Input: part model. Units: mm. Frame: model coordinates. A direction names the side the tool comes from. Give positions to 0.01 mm unless a question says otherwise; leave off trailing zeros. Loops run counter-clockwise (first coordinate to the right, second up) from the corner with the lowest first, then second, coordinate; pieces in that order, holes last. Notation, with made-up numbers: (51, -12) - (107, -12) arc R23 ccw to (107, 16) - close; hole circle Ø4 at (72, 40). An arc over 180 degrees is marked (long way). Answer as a JSON object with one key per item and string values. Group by question number.
(1) Section query A-A (z = -1.25). Return loops of the section in (x, y), plus the area to 3 significant figures.
(2) Section query B-B (x = 12). Return loops of the section in (y, z), plus the area to 3 significant figures.
(3) Mould query, pull axis X, two halves, no side actions, for faces 4 (the flat face through (-19.05, -3, -0.02)), 5 (the flat face through (12, -5, 0)), 6 (the cylindrical face through (19, -4, -4)), 7 (the cylindrical face through (-15, -1, 4)). Classes: +X half, -X half, draft (parallel to the pull), parting line (faces both ways), or undercut.
(4) Pin query (flat end, axial travel): P1, Ø0.9, axis at y = -2, z = -0.5, coming from the +X side; P2, Ø3.5, axis at y = -1, z = 0.5, coming from the -X side; P3, Ø5, axis at x = -13, z = 2, coming from the -Y side. Return the tip coordinate at first contact, or that it passes through.
(5) Access query for faces 1 (the flat face through (14.95, -3, -0.02)), 2 (the flat face through (0, -5, 0)), 3 (the flat face through (-19.5, -4, 0)). Directions: +Z, -Z, +X, -X, +Y, -Y. A direction counts if a zero-diameter tool reaches every point of the face in a straight line with its end or side. Return the directions, or none.
(6) Section query C-C (z = 2). Return loops of the section in (x, y).
(7) Section query D-D (x = -1.5). Return loops of the section in (y, z).
(8) Material intervals for L1, parallel to X at y = -1.25, z = -2.25; L2, parallel to Y at x = 7, z = 4.5; L3, parallel to X at y = -0.75, z = -3.25, sorted ascending.
```python
from build123d import *

# Parameters (mm, degrees)
BOSS_EXTRU_2_DEPTH      = 5
BOSS_EXTRU_7_DEPTH      = 7
ESQUISSE1_13_W          = 0.6
ESQUISSE1_13_H          = 2.5
ENL_V_MAT_EXTRU_3_DEPTH = 3
ESQUISSE1_16_W          = 0.6
ESQUISSE1_16_H          = 2.5
ENL_V_MAT_EXTRU_4_DEPTH = 3


with BuildPart() as part:
    # Esquisse1 → Boss.-Extru.2 (new body)
    with BuildSketch(Plane(origin=(0, 0, 0), x_dir=(1, 0, 0), z_dir=(0, 1, 0))):
        with BuildLine():
            Line((-17, -5), (17, -5))
            ThreePointArc((17, -5), (18.767766953, -4.267766953), (19.5, -2.5))
            Line((19.5, -2.5), (19.5, 2.5))
            ThreePointArc((19.5, 2.5), (18.767766953, 4.267766953), (17, 5))
            Line((17, 5), (-17, 5))
            ThreePointArc((-17, 5), (-18.767766953, 4.267766953), (-19.5, 2.5))
            Line((-19.5, 2.5), (-19.5, -2.5))
            ThreePointArc((-19.5, -2.5), (-18.767766953, -4.267766953), (-17, -5))
        make_face()
    extrude(amount=-BOSS_EXTRU_2_DEPTH)

    # Esquisse1_9 → Boss.-Extru.7 (add)
    with BuildSketch(Plane(origin=(0, 0, 0), x_dir=(1, 0, 0), z_dir=(0, 1, 0))):
        with BuildLine():
            ThreePointArc((-5, 0), (-3.535533906, -3.535533906), (0, -5))
            ThreePointArc((0, -5), (3.535533906, -3.535533906), (5, 0))
            Line((5, 0), (3.5, 0))
            ThreePointArc((3.5, 0), (0, -3.5), (-3.5, 0))
            Line((-3.5, 0), (-5, 0))
        make_face()
        with BuildLine():
            Line((3.5, 0), (5, 0))
            ThreePointArc((5, 0), (3.535533906, 3.535533906), (0, 5))
            ThreePointArc((0, 5), (-3.535533906, 3.535533906), (-5, 0))
            Line((-5, 0), (-3.5, 0))
            ThreePointArc((-3.5, 0), (0, 3.5), (3.5, 0))
        make_face()
    extrude(amount=-BOSS_EXTRU_7_DEPTH)

    # Esquisse1_13 → Enl_v. mat.-Extru.3 (cut)
    with BuildSketch(Plane(origin=(0, 0, 0), x_dir=(1, 0, 0), z_dir=(0, 1, 0))):
        with BuildLine():
            ThreePointArc((17, 5), (15.232233047, 4.267766953), (14.5, 2.5))
            Line((14.5, 2.5), (15.1, 2.5))
            ThreePointArc((15.1, 2.5), (15.656497116, 3.843502884), (17, 4.4))
            Line((17, 4.4), (17, 5))
        make_face()
        with BuildLine():
            ThreePointArc((19.5, 2.5), (18.767766953, 4.267766953), (17, 5))
            Line((17, 5), (17, 4.4))
            ThreePointArc((17, 4.4), (18.343502884, 3.843502884), (18.9, 2.5))
            Line((18.9, 2.5), (19.5, 2.5))
        make_face()
        with Locations((19.2, 1.25)):
            Rectangle(ESQUISSE1_13_W, ESQUISSE1_13_H)
        with Locations((19.2, -1.25)):
            Rectangle(ESQUISSE1_13_W, ESQUISSE1_13_H)
        with BuildLine():
            Line((17, -4.4), (17, -5))
            ThreePointArc((17, -5), (18.767766953, -4.267766953), (19.5, -2.5))
            Line((19.5, -2.5), (18.9, -2.5))
            ThreePointArc((18.9, -2.5), (18.343502884, -3.843502884), (17, -4.4))
        make_face()
        with BuildLine():
            ThreePointArc((14.5, -2.5), (15.232233047, -4.267766953), (17, -5))
            Line((17, -5), (17, -4.4))
            ThreePointArc((17, -4.4), (15.656497116, -3.843502884), (15.1, -2.5))
            Line((15.1, -2.5), (14.5, -2.5))
        make_face()
        with Locations((14.8, -1.25)):
            Rectangle(ESQUISSE1_13_W, ESQUISSE1_13_H)
        with Locations((14.8, 1.25)):
            Rectangle(ESQUISSE1_13_W, ESQUISSE1_13_H)
    extrude(amount=-ENL_V_MAT_EXTRU_3_DEPTH, mode=Mode.SUBTRACT)

    # Esquisse1_16 → Enl_v. mat.-Extru.4 (cut)
    with BuildSketch(Plane(origin=(0, 0, 0), x_dir=(1, 0, 0), z_dir=(0, 1, 0))):
        with BuildLine():
            ThreePointArc((-19.5, -2.5), (-18.767766953, -4.267766953), (-17, -5))
            Line((-17, -5), (-17, -4.4))
            ThreePointArc((-17, -4.4), (-18.343502884, -3.843502884), (-18.9, -2.5))
            Line((-18.9, -2.5), (-19.5, -2.5))
        make_face()
        with Locations((-19.2, -1.25)):
            Rectangle(ESQUISSE1_16_W, ESQUISSE1_16_H)
        with Locations((-19.2, 1.25)):
            Rectangle(ESQUISSE1_16_W, ESQUISSE1_16_H)
        with BuildLine():
            Line((-17, 4.4), (-17, 5))
            ThreePointArc((-17, 5), (-18.767766953, 4.267766953), (-19.5, 2.5))
            Line((-19.5, 2.5), (-18.9, 2.5))
            ThreePointArc((-18.9, 2.5), (-18.343502884, 3.843502884), (-17, 4.4))
        make_face()
        with BuildLine():
            Line((-15.1, 2.5), (-14.5, 2.5))
            ThreePointArc((-14.5, 2.5), (-15.232233047, 4.267766953), (-17, 5))
            Line((-17, 5), (-17, 4.4))
            ThreePointArc((-17, 4.4), (-15.656497116, 3.843502884), (-15.1, 2.5))
        make_face()
        with Locations((-14.8, 1.25)):
            Rectangle(ESQUISSE1_16_W, ESQUISSE1_16_H)
        with Locations((-14.8, -1.25)):
            Rectangle(ESQUISSE1_16_W, ESQUISSE1_16_H)
        with BuildLine():
            Line((-17, -4.4), (-17, -5))
            ThreePointArc((-17, -5), (-15.232233047, -4.267766953), (-14.5, -2.5))
            Line((-14.5, -2.5), (-15.1, -2.5))
            ThreePointArc((-15.1, -2.5), (-15.656497116, -3.843502884), (-17, -4.4))
        make_face()
    extrude(amount=-ENL_V_MAT_EXTRU_4_DEPTH, mode=Mode.SUBTRACT)


solid = part.part
```
Recorded:
{
 "1": {"outline": "(-19.5, -5) - (-4.84, -5) - (-4.84, -7) - (-3.27, -7) - (-3.27, -5) - (3.27, -5) - (3.27, -7) - (4.84, -7) - (4.84, -5) - (19.5, -5) - (19.5, -3) - (18.9, -3) - (18.9, 0) - (15.1, 0) - (15.1, -3) - (14.5, -3) - (14.5, 0) - (-14.5, 0) - (-14.5, -3) - (-15.1, -3) - (-15.1, 0) - (-18.9, 0) - (-18.9, -3) - (-19.5, -3) - close", "area": "194 mm^2"},
 "2": {"outline": "(-5, -5) - (0, -5) - (0, 5) - (-5, 5) - close", "area": "50.0 mm^2"},
 "3": {"face 4": "undercut", "face 5": "draft", "face 6": "+X half", "face 7": "undercut"},
 "4": {"P1": "stops at x = 18.9", "P2": "stops at x = -18.9", "P3": "stops at y = -5"},
 "5": {"face 1": "+Y", "face 2": "-Y", "face 3": "+Z, -Z, -X, +Y, -Y"},
 "6": {"outline": "(-19.5, -5) - (-4.58, -5) - (-4.58, -7) - (-2.87, -7) - (-2.87, -5) - (2.87, -5) - (2.87, -7) - (4.58, -7) - (4.58, -5) - (19.5, -5) - (19.5, -3) - (18.9, -3) - (18.9, 0) - (15.1, 0) - (15.1, -3) - (14.5, -3) - (14.5, 0) - (-14.5, 0) - (-14.5, -3) - (-15.1, -3) - (-15.1, 0) - (-18.9, 0) - (-18.9, -3) - (-19.5, -3) - close"},
 "7": {"outline": "(-7, -4.77) - (-5, -4.77) - (-5, -5) - (0, -5) - (0, 5) - (-5, 5) - (-5, 4.77) - (-7, 4.77) - (-7, 3.16) - (-5, 3.16) - (-5, -3.16) - (-7, -3.16) - close"},
 "8": {"L1": "x = -18.9 to -15.1, -14.5 to 14.5, 15.1 to 18.9", "L2": "y = -5 to 0", "L3": "x = -18.75 to -15.25, -14.62 to 14.62, 15.25 to 18.75"}
}
